Verification items for the finished model (mm, model axes). Face numbers are marked on the shaded views. A direction names the side the tool comes from. Round coordinates to 2 decimals unless told otherwise and drop trailing zeros. Write each loop counter-clockwise with the first axis right and the second up, starting at its lowest first coordinate (ties: lowest second). Pieces come first, ordered by that corner, then holes. Notation, with made-up numbers: (-16, -16) - (9, -16) arc R32 cw to (9, 22) - close; hole circle Ø9 at (47.5, 83.5). An arc over 180 degrees is marked (long way). Answer as a JSON object with one key per item and string values.
```python
from build123d import *

# Parameters (mm, degrees)
F1_DEPTH = 10


with BuildPart() as f1:
    # F0 (on Top) → F1 (new body)
    with BuildSketch(Plane.XY):
        with BuildLine():
            Line((0, 14), (0, 0))
            Line((0, 0), (5, 0))
            ThreePointArc((5, 0), (10.069501, 1.380246), (13.739571, 5.139969))
            ThreePointArc((13.739571, 5.139969), (20.513532, 11.226724), (29.598437, 11.858887))
            Line((29.598437, 11.858887), (44, 8))
            Line((44, 8), (60, 8))
            Line((60, 8), (65, 13))
            Line((65, 13), (65, 17))
            Line((65, 17), (50, 17))
            ThreePointArc((50, 17), (44.387514, 18.089572), (39.590389, 21.2))
            ThreePointArc((39.590389, 21.2), (36.392306, 23.273618), (32.650648, 24))
            Line((32.650648, 24), (10, 24))
            Line((10, 24), (0, 14))
        make_face()
    extrude(amount=F1_DEPTH)


solid = f1.part
```
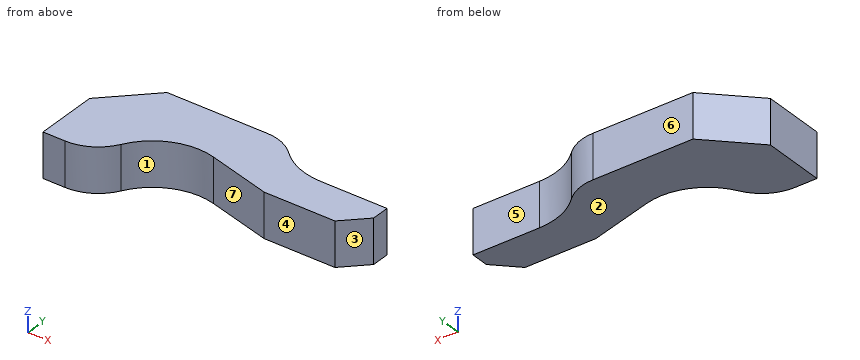
1. Cross-section at B-B (z = 5.5). Record the boundary of the cut face in (x, y), plus the area to 3 significant figures.
Completed:
{"outline": "(0, 0) - (5, 0) arc R10 ccw to (13.74, 5.14) arc R14 cw to (29.6, 11.86) - (44, 8) - (60, 8) - (65, 13) - (65, 17) - (50, 17) arc R15 cw to (39.59, 21.2) arc R10 ccw to (32.65, 24) - (10, 24) - (0, 14) - close", "area": "834 mm^2"}
2. Go/stop test with flat-tipped pins: pin 1 (4 mm diameter, centred on x = 50.5, z = 1.5, fed in from +Y); pin 2 (2 mm diameter, centred on y = 16, z = 5, fed in from -X). Record where each tip stops, or that it passes through.
Completed:
{"pin 1": "stops at y = 17.08", "pin 2": "stops at x = 1"}
3. Cross-section at A-A (y = 10.5). Record the boundary of the cut face in (x, z).
Completed:
{"outline": "(0, 0) - (19.04, 0) - (19.04, 10) - (0, 10) - close; (34.67, 0) - (62.5, 0) - (62.5, 10) - (34.67, 10) - close"}
4. Material ranges on probe 1 along X at (y, z) = (12.75, 4.5); probe 2 along X at (y, z) = (2.25, 2.25); probe 3 along Y at (x, z) = (18.5, 8.75), recorded low to high. Write a range as from..to.
Completed:
{"probe 1": "x = 0..64.75", "probe 2": "x = 0..11.32", "probe 3": "y = 10.17..24"}
5. Access from +Z, -Z, +X, -X, +Y, -Y to the whole of each face (thin tool, end or side, straight path). Record for the marked faces 4, 5, 6 and 7.
Completed:
{"face 4": "+Z, -Z, +X, -Y", "face 5": "+Z, -Z, +X, +Y", "face 6": "+Z, -Z, +X, -X, +Y", "face 7": "+Z, -Z, -Y"}
6. Mould release check, pull along X, two halves, no side actions. Record for the marked faces 1, 2 and 3: released by +X, released by -X, zero draft, split by the parting line, or undercut.
Completed:
{"face 1": "undercut", "face 2": "zero draft", "face 3": "released by +X"}
7. Cross-section at D-D (y = 19.75). Record the boundary of the cut face in (x, z).
Completed:
{"outline": "(5.75, 0) - (41.34, 0) - (41.34, 10) - (5.75, 10) - close"}
8. Cross-section at C-C (x = 57.5). Record the boundary of the cut face in (y, z).
Completed:
{"outline": "(8, 0) - (17, 0) - (17, 10) - (8, 10) - close"}
